CAD build for the part. Positions are in the model's coordinates, mm. A direction names the side the tool comes from. Give positions to 0.01 mm unless a question says otherwise; leave off trailing zeros. Loops run counter-clockwise (first coordinate to the right, second up) from the corner with the lowest first, then second, coordinate; pieces in that order, holes last. Notation, with made-up numbers: (-28.5, 70) -> (-4.5, 70) arc R15 cw to (-4.5, 79) -> close; hole circle Ø10 at (62, -29.75). An arc over 180 degrees is marked (long way). Use one line per item in the form item = value.
```python
from build123d import *

# Parameters (mm, degrees)
SKETCH1_W                = 17.8
SKETCH1_H                = 6.2
BOSS_EXTRUDE1_DEPTH      = 5.4
SHELL1_T                 = -1.2
SKETCH2_W                = 6
SKETCH2_H                = 4.2
REVOLVE1_DEPTH           = 8
SKETCH5_W                = 1.864108749
SKETCH5_H                = 2.6
CUT_EXTRUDE1_DEPTH       = 5.4
SKETCH6_W                = 5.2
SKETCH6_H                = 1.6
CUT_EXTRUDE2_DEPTH       = 2.7
SKETCH7_R                = 1.5
BOSS_EXTRUDE2_DEPTH      = 3.8
SKETCH9_W                = 5.3
SKETCH9_H                = 2.5
CUT_EXTRUDE3_DEPTH       = 5
SKETCH12_W               = 1.4
SKETCH12_H               = 3
CUT_EXTRUDE4_DEPTH       = 5
BOSS_EXTRUDE5_DEPTH      = 1.3
CHAMFER1_SIZE            = 0.5
CHAMFER1_OF_MIRROR1_SIZE = 0.5
SKETCH13_W               = 2.2
SKETCH13_H               = 1.8
BOSS_EXTRUDE6_DEPTH      = 1.2


# Read off the part's stored shape, not the designer's step: Revolve1
with BuildPart() as part:
    # Sketch1 → Boss-Extrude1 (new body)
    with BuildSketch(Plane(origin=(0, 0, 0), x_dir=(1, 0, 0), z_dir=(0, 1, 0))):
        Rectangle(SKETCH1_W, SKETCH1_H)
    extrude(amount=BOSS_EXTRUDE1_DEPTH)

    # Shell1
    shell1_openings = [part.faces().sort_by_distance(p)[0] for p in [
        (0, 2.7, 3.1),
    ]]
    offset(amount=SHELL1_T, openings=shell1_openings, kind=Kind.INTERSECTION)

    # Sketch2 → Cut-Revolve1 (revolve, cut)
    with BuildSketch(Plane.XY.offset(3.1)):
        with Locations((3, 3.3)):
            Rectangle(SKETCH2_W, SKETCH2_H)
    revolve(axis=Axis((0, 1.2, 3.1), (0, 1, 0)), mode=Mode.SUBTRACT)

    # Revolve1 outline → Revolve1 (add)
    with BuildSketch(Plane(origin=(0, 0, 0), x_dir=(1, 0, 0), z_dir=(0, 1, 0))):
        with BuildLine():
            Line((-5.180733539, 1.9), (-3.31662479, 1.9))
            ThreePointArc((-3.31662479, 1.9), (0, 2.9), (3.31662479, 1.9))
            Line((3.31662479, 1.9), (5.180733539, 1.9))
            ThreePointArc((5.180733539, 1.9), (0, 4.1), (-5.180733539, 1.9))
        make_face()
    extrude(amount=REVOLVE1_DEPTH)

    # Sketch5 → Cut-Extrude1 (cut)
    with BuildSketch(Plane.XY.offset(-1.9)):
        with Locations((-4.248679165, 6.7)):
            Rectangle(SKETCH5_W, SKETCH5_H)
        with Locations((4.248679165, 6.7)):
            Rectangle(SKETCH5_W, SKETCH5_H)
    extrude(amount=-CUT_EXTRUDE1_DEPTH, mode=Mode.SUBTRACT)

    # Sketch6 → Cut-Extrude2 (cut, symmetric)
    with BuildSketch(Plane(origin=(0, 0, -3.1), x_dir=(-1, 0, 0), z_dir=(0, 0, -1))):
        with Locations((0, 2)):
            Rectangle(SKETCH6_W, SKETCH6_H)
    extrude(amount=CUT_EXTRUDE2_DEPTH, both=True, mode=Mode.SUBTRACT)

    # Sketch7 → Boss-Extrude2 (add)
    with BuildSketch(Plane(origin=(0, 0, -3.1), x_dir=(-1, 0, 0), z_dir=(0, 0, -1))):
        with Locations(Location((6.1, 3.4, 0), (0, 0, 180))):
            Circle(SKETCH7_R)
        with Locations(Location((-6.1, 3.4, 0), (0, 0, 180))):
            Circle(SKETCH7_R)
    extrude(amount=BOSS_EXTRUDE2_DEPTH)

    # Sketch9 → Cut-Extrude3 (cut, symmetric)
    with BuildSketch(Plane(origin=(0, 1.2, 0), x_dir=(1, 0, 0), z_dir=(0, 1, 0))):
        with Locations((0, -1.85)):
            Rectangle(SKETCH9_W, SKETCH9_H)
    extrude(amount=CUT_EXTRUDE3_DEPTH, both=True, mode=Mode.SUBTRACT)

    # Sketch12 → Cut-Extrude4 (cut, symmetric)
    with BuildSketch(Plane(origin=(8.9, 0, 0), x_dir=(0, 0, -1), z_dir=(1, 0, 0))):
        with Locations((-2.4, 2.7)):
            Rectangle(SKETCH12_W, SKETCH12_H)
    cut_extrude4 = extrude(amount=CUT_EXTRUDE4_DEPTH, both=True, mode=Mode.SUBTRACT)

    # Sketch11 → Boss-Extrude5 (add)
    with BuildSketch(Plane(origin=(8.9, 0, 0), x_dir=(0, 0, -1), z_dir=(1, 0, 0))):
        Polygon((-1, 0), (-1, 5.4), (-3.1, 5.4), (-3.1, 4.2), (-1.7, 4.2), (-1.7, 1.2), (-3.1, 1.2), (-3.1, 0), align=None)
        Polygon((-3.1, 4.2), (-3.1, 5.4), (-4.3, 5.4), (-4.3, 0), (-3.1, 0), (-3.1, 1.2), align=None)
    boss_extrude5 = extrude(amount=BOSS_EXTRUDE5_DEPTH)

    # Chamfer1
    chamfer1_edges = [part.edges().sort_by_distance(p)[0] for p in [
        (10.2, 2.7, 1),
    ]]
    chamfer(chamfer1_edges, length=CHAMFER1_SIZE)

    # Mirror1: Cut-Extrude4, Boss-Extrude5 across plane
    add(cut_extrude4.mirror(Plane(origin=(0, 0, 0), x_dir=(0, 0, 1), z_dir=(1, 0, 0))), mode=Mode.SUBTRACT)
    add(boss_extrude5.mirror(Plane(origin=(0, 0, 0), x_dir=(0, 0, 1), z_dir=(1, 0, 0))))

    # Chamfer1 of Mirror1
    chamfer1_of_mirror1_edges = [part.edges().sort_by_distance(p)[0] for p in [
        (-10.2, 2.7, 1),
    ]]
    chamfer(chamfer1_of_mirror1_edges, length=CHAMFER1_OF_MIRROR1_SIZE)

    # Sketch13 → Boss-Extrude6 (add)
    with BuildSketch(Plane(origin=(0, 1.2, 0), x_dir=(1, 0, 0), z_dir=(0, 1, 0))):
        with Locations((0, -1.5)):
            Rectangle(SKETCH13_W, SKETCH13_H)
    extrude(amount=-BOSS_EXTRUDE6_DEPTH)


solid = part.part
```
1. Cut at B-B, the plane y = 1.5. State how many separate pieces and enclosed holes the cut face has, then the cut area to 3 significant figures.
Result sheet:
separate_pieces = 4
enclosed_holes = 0
area = 28.7 mm^2
2. Mould opens along Z. For faces 5 (the flat face through (7, 2, -3.1)), 6 (the flat face through (0, 1, 2.4)), 7 (the flat face through (-10, 3, 3.1)) say: pulls with the +Z half, pulls with the -Z half, needs draft (parallel to the pull), parting line crosses it, or undercut.
Result sheet:
face_5 = pulls with the -Z half
face_6 = pulls with the +Z half
face_7 = undercut
3. Cut at A-A, the plane z = 3.5. Write the cut outline in (x, y).
Result sheet:
outline = (-10.2, 0) -> (-8.9, 0) -> (-8.9, 5.4) -> (-10.2, 5.4) -> close; (8.9, 0) -> (10.2, 0) -> (10.2, 5.4) -> (8.9, 5.4) -> close
4. Drill centre lines: line 1 (X direction, y = 2, z = -1); line 2 (Z direction, x = -3.75, y = 0.5); line 3 (Y direction, x = 2.75, z = -2). Where is each one in solid material? Low to high.
Result sheet:
line_1 = -8.9 to -7.7, 7.7 to 8.9
line_2 = -3.1 to 3.1
line_3 = 0 to 1.2
5. Drop flat-ended pins along their axis: P1, Ø4, axis at x = 6, y = 1, coming from the +Z side; P2, Ø0.6, axis at x = 9.5, y = 3.5, coming from the -Z side; P3, Ø4, axis at x = 2, z = 0.5, coming from the +Y side. Give the stop position or say it passes through.
Result sheet:
P1 = 3.1
P2 = 1
P3 = 1.2
6. Cut at C-C, the plane x = 0. Write the cut outline in (y, z).
Result sheet:
outline = (0, -4.1) -> (1.2, -4.1) -> (1.2, 2.4) -> (0, 2.4) -> close; (2.8, -4.1) -> (8, -4.1) -> (8, -2.9) -> (2.8, -2.9) -> close
7. Tool access for faces 1 (the flat face through (-8.9, 3, -1)), 2 (the flat face through (7, 4.2, 1)), 3 (the flat face through (-1.1, 1, 2)), 4 (the flat face through (10, 3, 3.1)): list every direction of +Z, -Z, +X, -X, +Y, -Y with a clear straight run to the whole face (end or side of a thin tool).
Result sheet:
face_1 = -Z, -X, +Y, -Y
face_2 = none
face_3 = +Z, +Y, -Y
face_4 = +X, -X
